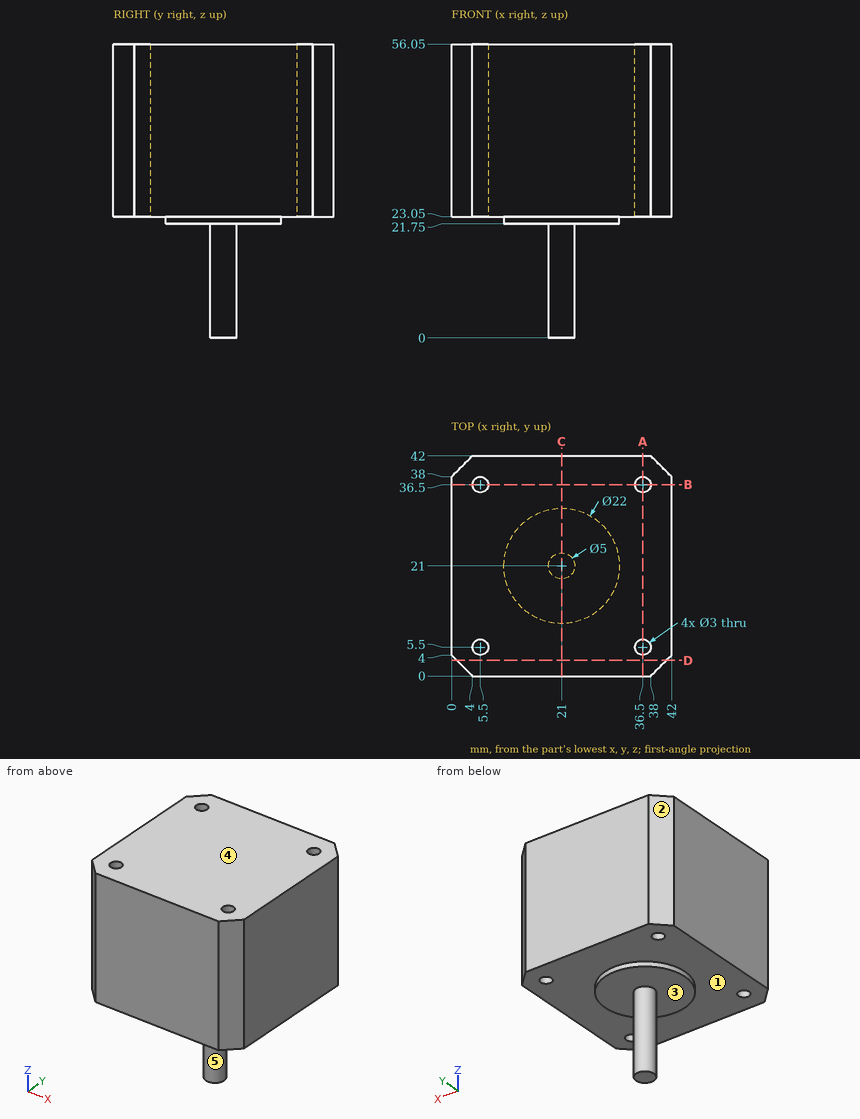
The drawing under review shows one solid part. Ordinate dimensions are in mm from its lowest x, y, z. A direction names the side the tool comes from. Round coordinates to 2 decimals unless told otherwise and drop trailing zeros. Write each loop counter-clockwise with the first axis right and the second up, starting at its lowest first coordinate (ties: lowest second). Pieces come first, ordered by that corner, then holes. Notation, with made-up numbers: (-9, 56) - (20, 56) arc R19 ccw to (20, 89) - close; hole circle Ø1 at (83.5, -32.5). An arc over 180 degrees is marked (long way). One line per question, with ' | ' between items.
Item 1: For P1, Ø1.5, axis at x = 19, y = 12.5, coming from the -Z side; P2, Ø5, axis at x = 5.5, y = 5.5, coming from the +Z side; P3, Ø1.8, axis at x = 5.5, y = 36.5, coming from the -Z side; P4, Ø1, axis at x = 36, y = 7, coming from the -Z side, all flat-tipped, find the tip position at first contact; note any pin that passes through.
Resolved:
P1: stops at z = 21.75 | P2: stops at z = 56.05 | P3: passes through | P4: stops at z = 23.05
Item 2: Add section D-D, the plane y = 3. Give the boundary of the cut face in (x, z).
Resolved:
outline: (1, 23.05) - (41, 23.05) - (41, 56.05) - (1, 56.05) - close
Item 3: Add section C-C, the plane x = 21. Give the boundary of the cut face in (y, z), then the cut area to 3 significant figures.
Resolved:
outline: (0, 23.05) - (10, 23.05) - (10, 21.75) - (18.5, 21.75) - (18.5, 0) - (23.5, 0) - (23.5, 21.75) - (32, 21.75) - (32, 23.05) - (42, 23.05) - (42, 56.05) - (0, 56.05) - close | area: 1,520 mm2
Item 4: For the marked faces 1 and 2, list the 3-axis set-ups (+Z, -Z, +X, -X, +Y, -Y) from which the entire face can be reached by the end or side of a thin tool; tool diameter is ignored.
Resolved:
face 1: -Z | face 2: +Z, -Z, -X, +Y
Item 5: The part is to be moulded in two halves that separate along Z. For the marked faces 3, 4 and 5, say which applies: pulls with the +Z half, pulls with the -Z half, needs draft (parallel to the pull), parting line crosses it, or undercut.
Resolved:
face 3: pulls with the -Z half | face 4: pulls with the +Z half | face 5: needs draft
Item 6: Add section A-A, the plane x = 36.5. Give the boundary of the cut face in (y, z).
Resolved:
outline: (0, 23.05) - (4, 23.05) - (4, 56.05) - (0, 56.05) - close; (7, 23.05) - (35, 23.05) - (35, 56.05) - (7, 56.05) - close; (38, 23.05) - (42, 23.05) - (42, 56.05) - (38, 56.05) - close
Item 7: To check wall thickness, follow probe 1 along Y at (x, z) = (5.5, 43.5); probe 2 along Z at (x, y) = (26, 38); probe 3 along X at (y, z) = (35.5, 26). State the ranges of each line that lie inside material, in increasing order.
Resolved:
probe 1: y = 0 to 4, 7 to 35, 38 to 42 | probe 2: z = 23.05 to 56.05 | probe 3: x = 0 to 4.38, 6.62 to 35.38, 37.62 to 42
